Source: CAD feature listing. Evaluate the final solid. Frame: model axes, mm. A direction names the side the tool comes from. Round coordinates to 2 decimals unless told otherwise and drop trailing zeros. Order: outer loops, then holes, each group sorted by start corner. A loop starts at its lowest first (then second) coordinate and runs counter-clockwise, first axis right, second up. Notation, with made-up numbers: (67.25, 16) - (74.25, 16) arc R27 ccw to (74.25, 37) - close; hole circle Ø3 at (-19.75, -7.5). An arc over 180 degrees is marked (long way). Use one line per item in the form item = value. Start each with the question number.
Q1. Ray query, line 1 (Y direction, x = 85.75, z = -11); line 2 (Y direction, x = 41.75, z = 0.85); line 3 (Y direction, x = 116, z = -7.75). Return the intervals inside material, ascending. Write a range as [from, to].
Q2. Draft query along Y for faces 1 (the flat face through (2, 3, 0)), 2 (the flat face through (87, 11, -2)), 3 (the flat face through (61, 51, 15)), 4 (the cylindrical face through (31.25, 13.93, -0.79)). Return one class per face: released by +Y, released by -Y, zero draft, split by the parting line, or undercut.
Q3. Cut plane B-B, the plane z = 9.5. Give the number of separate pieces and of enclosed holes in the cut face, and give its area (3 significant figures).
Q4. Cut plane C-C, the plane x = 45.75. Return the cut outline in (y, z).
Q5. Cut plane A-A, the plane x = 111.5. Return the cut outline in (y, z).
Q6. Pin query (flat end, axial travel): pin 1 Ø8 at (x, y) = (84.5, 45.5) entering from +Z; pin 2 Ø2.5 at (x, y) = (64.5, 45) entering from -Z. Return the tip coordinate at first contact, or that it passes through.
Q7. Set-up query: faces 5 (the flat face through (43, 11, -2)), 6 (the flat face through (122, 2.5, 0.7)), 7 (the flat face through (62, 12.5, -1)), 8 (the cylindrical face through (2.5, 42.1, 0.7)). Return all of +Z, -Z, +X, -X, +Y, -Y with unobstructed straight access to the full face (end or side cutting, diameter ignored); none if empty.
Solid Edge part; units mm, degrees
sketch "Sketch1" plane through (0, 0, 0) normal (0, 0, 1) x (1, 0, 0)
  line L0 (0, 0) -> (124.5, 0)
  line L1 (124.5, 0) -> (124.5, 54)
  line L2 (124.5, 54) -> (0, 54)
  line L3 (0, 54) -> (0, 0)
extrude "Protrusion1" add sketch "Sketch1" along normal up to vertex (15 mm away) and the other way up to vertex (17.5 mm away)
chamfer "Chamfer1" distance 5 angle 45 4 edges at (0, 0, -1.25) (124.5, 0, -1.25) (124.5, 54, -1.25) (0, 54, -1.25)
sketch "Sketch2" plane through (62.25, 27, 15) normal (0, 0, 1) x (1, 0, 0)
  line L0 (-56.25, 11.5) -> (-40.25, 11.5)
  line L1 (-40.25, 18.5) -> (-56.25, 18.5)
  arc A0 (-40.25, 18.5) -> (-40.25, 11.5) centre (-40.25, 15) cw
  arc A1 (-56.25, 11.5) -> (-56.25, 18.5) centre (-56.25, 15) cw
extrude "Cutout1" cut sketch "Sketch2" against normal through all
pattern_linear "Pattern1" count 2 spacing 96.5 along (1, 0, 0) count 2 spacing 30 along (0, -1, 0) of "Cutout1"
sketch "Sketch3" plane through (62.25, 27, 15) normal (0, 0, 1) x (1, 0, 0)
  line L0 (32.5, 14.5) -> (-32.5, 14.5)
  line L1 (-32.5, 14.5) -> (-32.5, -14.5)
  line L2 (-32.5, -14.5) -> (32.5, -14.5)
  line L3 (32.5, -14.5) -> (32.5, 14.5)
extrude "Cutout2" cut sketch "Sketch3" against normal through all
sketch "Sketch4" plane through (62.25, 27, 15) normal (0, 0, 1) x (1, 0, 0)
  line L0 (32.5, 23) -> (-32.5, 23)
  line L1 (-32.5, 23) -> (-32.5, -23)
  line L2 (-32.5, -23) -> (32.5, -23)
  line L3 (32.5, -23) -> (32.5, 23)
extrude "VaciadoExtruido_3" cut sketch "Sketch4" against normal blind 13
fillet "Redondeo_1" radius 5 8 edges at (29.75, 50, 8.5) (94.75, 50, 8.5) (94.75, 4, 8.5) (94.75, 12.5, -7.75) (94.75, 41.5, -7.75) (29.75, 41.5, -7.75) (29.75, 4, 8.5) (29.75, 12.5, -7.75)
sketch "Sketch5" plane through (62.25, 27, -17.5) normal (0, 0, -1) x (-1, 0, 0)
  line L0 (-32.5, 23) -> (-32.5, -23)
  line L1 (-32.5, -23) -> (32.5, -23)
  line L2 (32.5, -23) -> (32.5, 23)
  line L3 (32.5, 23) -> (-32.5, 23)
extrude "Protrusion2" add sketch "Sketch5" against normal up to vertex (14 mm away)
sketch "Sketch6" plane through (62.25, 27, -17.5) normal (0, 0, -1) x (-1, 0, 0)
  circle A0 centre (16.5, 0) radius 8.5
extrude "Cutout3" cut sketch "Sketch6" against normal up to vertex (14 mm away)
hole "Agujero_1" at (41.75, 9.7, 2) direction (0, 0, -1) diameter 3 end through all
hole "Hole1" at (63.75, 9.7, 2) direction (0, 0, -1) diameter 3 end through all
hole "Hole2" at (85.75, 9.7, 2) direction (0, 0, -1) diameter 3 end through all
hole "Hole3" at (41.75, 44.3, 2) direction (0, 0, -1) diameter 3 end through all
hole "Hole4" at (63.75, 44.3, 2) direction (0, 0, -1) diameter 3 end through all
hole "Hole5" at (85.75, 44.3, 2) direction (0, 0, -1) diameter 3 end through all
sketch "Sketch7" plane through (14, 27, -14) normal (0, 0, -1) x (-1, 0, 0)
  line L0 (15.0837, -36.0096) -> (-114.5837, -36.0096)
  line L1 (-114.5837, -36.0096) -> (-114.5837, 36.0096)
  line L2 (-114.5837, 36.0096) -> (15.0837, 36.0096)
  line L3 (15.0837, 36.0096) -> (15.0837, -36.0096)
extrude "VaciadoExtruido_8" cut sketch "Sketch7" along normal through all
hole "Agujero_7" at (41.75, 9.7, -14) direction (0, 0, 1) diameter 3 end up to next counterbore diameter 5 counterbore depth 12
hole "Hole6" at (63.75, 9.7, -14) direction (0, 0, 1) diameter 3 end up to next counterbore diameter 5 counterbore depth 12
hole "Hole7" at (85.75, 9.7, -14) direction (0, 0, 1) diameter 3 end up to next counterbore diameter 5 counterbore depth 12
hole "Hole8" at (41.75, 44.3, -14) direction (0, 0, 1) diameter 3 end up to next counterbore diameter 5 counterbore depth 12
hole "Hole9" at (63.75, 44.3, -14) direction (0, 0, 1) diameter 3 end up to next counterbore diameter 5 counterbore depth 12
hole "Hole10" at (85.75, 44.3, -14) direction (0, 0, 1) diameter 3 end up to next counterbore diameter 5 counterbore depth 12
sketch "Sketch8" plane through (62.25, 27, -3.5) normal (0, 0, 1) x (0, -1, 0)
  circle A0 centre (0, -16.5) radius 11.5
extrude "VaciadoExtruido_9" cut sketch "Sketch8" against normal blind 1.3
properties part number "1976-1300-002" material "Aluminio, 7075-T6"
Completed:
q1.line_1 = [0, 7.2], [12.2, 41.8], [46.8, 54]
q1.line_2 = [0, 8.2], [11.2, 12.5], [41.5, 42.8], [45.8, 54]
q1.line_3 = [0, 8.5], [15.5, 38.5], [45.5, 54]
q2.face_1 = released by -Y
q2.face_2 = undercut
q2.face_3 = zero draft
q2.face_4 = undercut
q3.separate_pieces = 1
q3.enclosed_holes = 5
q3.area = 3,100 mm2
q4.outline = (0, -14) - (18.5, -14) - (18.5, -4.8) - (15.5, -4.8) - (15.5, -3.5) - (12.5, -3.5) - (12.5, 2) - (4, 2) - (4, 15) - (0, 15) - close; (35.5, -14) - (54, -14) - (54, 15) - (50, 15) - (50, 2) - (41.5, 2) - (41.5, -3.5) - (38.5, -3.5) - (38.5, -4.8) - (35.5, -4.8) - close
q5.outline = (0, -14) - (8.5, -14) - (8.5, 15) - (0, 15) - close; (15.5, -14) - (38.5, -14) - (38.5, 15) - (15.5, 15) - close; (45.5, -14) - (54, -14) - (54, 15) - (45.5, 15) - close
q6.pin_1 = 2
q6.pin_2 = -2
q7.face_5 = -Z
q7.face_6 = +Z, -Z, +X, -Y
q7.face_7 = +Z
q7.face_8 = +Z, -Z
